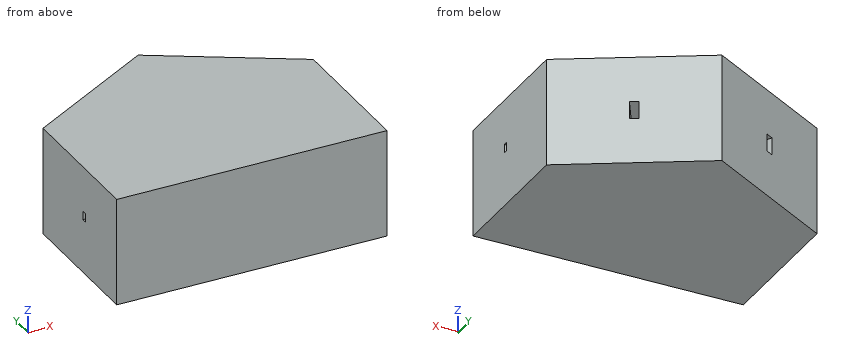
from build123d import *

# Parameters (mm, degrees)
F0_W     = 24.15
F0_H     = 11.7
F1_DEPTH = 9.65
F2_W     = 0.775
F2_H     = 1.55
F3_DEPTH = 48.3
F4_W     = 1.55
F4_H     = 1.55
F5_DEPTH = 10
F6_W     = 1.55
F6_H     = 1.55
F7_DEPTH = 10


with BuildPart() as f1:
    # F0 (on Top) → F1 (new body, symmetric)
    with BuildSketch(Plane.XY):
        Polygon((-24.15, 11.7), (0, 11.7), (-12.075, 32.6145135014), (-24.15, 25.6430090009), align=None)
        with Locations((-12.075, 5.85)):
            Rectangle(F0_W, F0_H)
        with Locations((12.075, 5.85)):
            Rectangle(F0_W, F0_H)
        Polygon((12.075, 32.6145135014), (0, 11.7), (24.15, 11.7), (24.15, 25.6430090009), align=None)
        Polygon((-12.075, 32.6145135014), (0, 11.7), (12.075, 32.6145135014), (0, 39.5860180019), align=None)
    extrude(amount=F1_DEPTH, both=True)

    # F2 (on face) → F3 (cut)
    with BuildSketch(Plane(origin=(-24.15, 0, 0), x_dir=(0, -1, 0), z_dir=(-1, 0, 0))):
        with Locations((-11.3125, 0.775)):
            Rectangle(F2_W, F2_H)
    extrude(amount=-F3_DEPTH, mode=Mode.SUBTRACT)

    # F4 (on face) → F5 (cut)
    with BuildSketch(Plane(origin=(17.1412486121, 29.6895135014, 0), x_dir=(-0.8660254038, 0.5, 0), z_dir=(0.5, 0.8660254038, 0))):
        with Locations((5.85, 0.775)):
            Rectangle(F4_W, F4_H)
        with Locations((5.85, -0.775)):
            Rectangle(F4_W, F4_H)
    extrude(amount=-F5_DEPTH, mode=Mode.SUBTRACT)

    # F6 (on face) → F7 (cut)
    with BuildSketch(Plane(origin=(-17.1412486121, 29.6895135014, 0), x_dir=(-0.8660254038, -0.5, 0), z_dir=(-0.5, 0.8660254038, 0))):
        with Locations((-5.85, -0.775)):
            Rectangle(F6_W, F6_H)
        with Locations((-5.85, 0.775)):
            Rectangle(F6_W, F6_H)
    extrude(amount=-F7_DEPTH, mode=Mode.SUBTRACT)


solid = f1.part
The model under review builds one solid part; all positions refer to its coordinate system, in mm. Round coordinates to 2 decimals unless told otherwise and drop trailing zeros. Write each loop counter-clockwise with the first axis right and the second up, starting at its lowest first coordinate (ties: lowest second). Pieces come first, ordered by that corner, then holes. Notation, with made-up numbers: (46, -36) -> (95, -36) arc R6 cw to (95, -26) -> close; hole circle Ø1 at (6.25, 24.5). An arc over 180 degrees is marked (long way). Answer as a JSON object with one key per item and string values.
1. Clearance check with flat-ended pins moving along their axes: pin 1 (1.7 mm diameter, centred on x = -9.5, z = 0.5, fed in from +Y); pin 2 (2 mm diameter, centred on y = 31.5, z = -0.5, fed in from -X); pin 3 (3 mm diameter, centred on x = 16, z = -5, fed in from -Y); pin 4 (5 mm diameter, centred on x = 4, z = -2, fed in from +Y). State where each tip first meets the part, or that it passes through.
Results found:
{"pin 1": "stops at y = 34.59", "pin 2": "stops at x = -15.74", "pin 3": "stops at y = 0", "pin 4": "stops at y = 38.72"}
2. We need section A-A on z = -0.75. State the section outline as (x, y) points, and give its area (3 significant figures).
Results found:
{"outline": "(-24.15, 0) -> (24.15, 0) -> (24.15, 25.64) -> (12.75, 32.23) -> (7.75, 23.57) -> (6.4, 24.34) -> (11.4, 33) -> (0, 39.59) -> (-11.4, 33) -> (-6.4, 24.34) -> (-7.75, 23.57) -> (-12.75, 32.23) -> (-24.15, 25.64) -> close", "area": "1,540 mm^2"}
3. To check wall thickness, follow line 1 along Z through (x, y) = (-2.5, 11); line 2 along X through (y, z) = (31, 1.5); line 3 along Y through (x, z) = (-19, -2.5). State the ranges of each line that lie inside material, in increasing order.
Results found:
{"line 1": "z = -9.65 to 0, 1.55 to 9.65", "line 2": "x = -14.87 to -12.04, -10.25 to 10.25, 12.04 to 14.87", "line 3": "y = 0 to 28.62"}
4. We need section B-B on x = 5. State the section outline as (y, z) points (3 decimals).
Results found:
{"outline": "(0, -9.65) -> (36.699, -9.65) -> (36.699, 9.65) -> (0, 9.65) -> close; hole (10.925, 0) -> (11.7, 0) -> (11.7, 1.55) -> (10.925, 1.55) -> close"}
5. We need section D-D on x = -18. State the section outline as (y, z) points (3 decimals).
Results found:
{"outline": "(0, -9.65) -> (29.194, -9.65) -> (29.194, 9.65) -> (0, 9.65) -> close; hole (10.925, 0) -> (11.7, 0) -> (11.7, 1.55) -> (10.925, 1.55) -> close"}
6. We need section C-C on y = 26.5. State the section outline as (x, z) points, and give its area (3 significant figures).
Results found:
{"outline": "(-22.67, -9.65) -> (22.67, -9.65) -> (22.67, 9.65) -> (-22.67, 9.65) -> close; hole (-9.44, -1.55) -> (-7.65, -1.55) -> (-7.65, 1.55) -> (-9.44, 1.55) -> close; hole (7.65, -1.55) -> (9.44, -1.55) -> (9.44, 1.55) -> (7.65, 1.55) -> close", "area": "864 mm^2"}
